from build123d import *

# Parameters (mm, degrees)
SKETCH1_R           = 59
BOSS_EXTRUDE1_DEPTH = 3
SKETCH3_R           = 51.75
BOSS_EXTRUDE2_DEPTH = 10
SKETCH4_R           = 50
CUT_EXTRUDE2_DEPTH  = 10
SCALE1_SCALE        = 0.5
SKETCH5_R           = 7.5
CUT_EXTRUDE3_DEPTH  = 15
SKETCH6_R           = 7.5
CUT_EXTRUDE4_DEPTH  = 15
SKETCH7_R           = 7.5
CUT_EXTRUDE5_DEPTH  = 15
SKETCH8_W           = 15
SKETCH8_H           = 16.086629849
CUT_EXTRUDE6_DEPTH  = 15


with BuildPart() as part:
    # Sketch1 → Boss-Extrude1 (new body)
    with BuildSketch(Plane(origin=(0, 0, 0), x_dir=(1, 0, 0), z_dir=(0, 1, 0))):
        with Locations(Location((0, 0, 0), (0, 0, 270))):
            Circle(SKETCH1_R)
    extrude(amount=BOSS_EXTRUDE1_DEPTH)

    # Sketch3 → Boss-Extrude2 (add)
    with BuildSketch(Plane(origin=(0, 3, 0), x_dir=(1, 0, 0), z_dir=(0, 1, 0))):
        with Locations(Location((0, 0, 0), (0, 0, 270))):
            Circle(SKETCH3_R)
    extrude(amount=BOSS_EXTRUDE2_DEPTH)

    # Sketch4 → Cut-Extrude2 (cut)
    with BuildSketch(Plane(origin=(0, 13, 0), x_dir=(1, 0, 0), z_dir=(0, 1, 0))):
        with Locations(Location((0, 0, 0), (0, 0, 270))):
            Circle(SKETCH4_R)
    extrude(amount=-CUT_EXTRUDE2_DEPTH, mode=Mode.SUBTRACT)


with BuildPart() as part_1:
    # Scale1: scaled about (0, 2.446860076, 0)
    add(part.part.scale(SCALE1_SCALE).moved(Location((0, 1.223430038, 0))))

    # Sketch5 → Cut-Extrude3 (cut)
    with BuildSketch(Plane(origin=(0, 2.723430038, 0), x_dir=(1, 0, 0), z_dir=(0, 1, 0))):
        with Locations(Location((0, -17.548132192, 0), (0, 0, 270))):
            Circle(SKETCH5_R)
    extrude(amount=-CUT_EXTRUDE3_DEPTH, mode=Mode.SUBTRACT)

    # Sketch6 → Cut-Extrude4 (cut)
    with BuildSketch(Plane(origin=(0, 7.723430038, 0), x_dir=(1, 0, 0), z_dir=(0, 1, 0))):
        with Locations((0, -25.513831206)):
            Circle(SKETCH6_R)
    extrude(amount=-CUT_EXTRUDE4_DEPTH, mode=Mode.SUBTRACT)

    # Sketch7 → Cut-Extrude5 (cut)
    with BuildSketch(Plane(origin=(0, 7.723430038, 0), x_dir=(1, 0, 0), z_dir=(0, 1, 0))):
        with Locations((0, -20.692487066)):
            Circle(SKETCH7_R)
    extrude(amount=-CUT_EXTRUDE5_DEPTH, mode=Mode.SUBTRACT)

    # Sketch8 → Cut-Extrude6 (cut)
    with BuildSketch(Plane(origin=(0, 2.723430038, 0), x_dir=(1, 0, 0), z_dir=(0, 1, 0))):
        with Locations((0, -25.591447116)):
            Rectangle(SKETCH8_W, SKETCH8_H)
    extrude(amount=-CUT_EXTRUDE6_DEPTH, mode=Mode.SUBTRACT)


solid = part_1.part
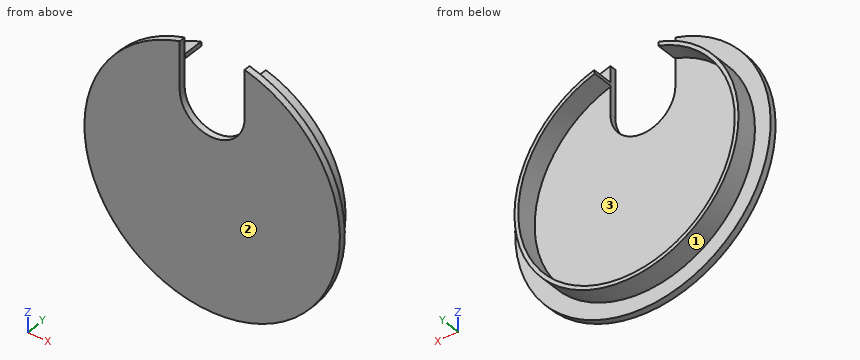
Input: part model. Units: mm. Frame: model coordinates. Face numbers are marked on the shaded views. Give positions to 0.01 mm unless a question says otherwise; leave off trailing zeros. Loops run counter-clockwise (first coordinate to the right, second up) from the corner with the lowest first, then second, coordinate; pieces in that order, holes last. Notation, with made-up numbers: M -35,10.5 L -29,10.5 A30 ccw -29,45.5 Z; hole C 57,85 d1. An arc over 180 degrees is marked long. Use one line per item in the form item = value.
1. Section query B-B, the plane x = -21. Return the cut outline in (y, z).
Numbers:
outline = M 1.22,-20.72 L 2.72,-20.72 L 2.72,-15.12 L 7.72,-15.12 L 7.72,-13.56 L 2.72,-13.56 L 2.72,13.56 L 7.72,13.56 L 7.72,15.12 L 2.72,15.12 L 2.72,20.72 L 1.22,20.72 Z
2. Section query A-A, the plane z = 12. Return the cut outline in (x, y), and give its area (3 significant figures).
Numbers:
outline = M -26.95,1.22 L -5.05,1.22 L -5.05,2.72 L -21.93,2.72 L -21.93,7.72 L -22.92,7.72 L -22.92,2.72 L -26.95,2.72 Z; M 5.05,1.22 L 26.95,1.22 L 26.95,2.72 L 22.92,2.72 L 22.92,7.72 L 21.93,7.72 L 21.93,2.72 L 5.05,2.72 Z
area = 75.6 mm²
3. Section query D-D, the plane y = 5. Return the cut outline in (x, z) (3 decimals).
Numbers:
outline = M -7.464,24.775 A25.875 ccw long 7.464,24.775 A7.5 cw 7.325,23.903 A25 cw long -7.325,23.903 A7.5 cw Z
4. First-contact query: pin 1 (1.5 mm diameter, centred on x = 11.5, y = 6, fed in from -Z); pin 2 (17.5 mm diameter, centred on x = 3, z = 14, fed in from +Y); pin 3 (1 mm diameter, centred on y = 5.5, z = 6, fed in from +X). Flat tips, straight axial feed; report the tip coordinate or a pass-through.
Numbers:
pin_1 = -23.54
pin_2 = 2.72
pin_3 = 25.28
5. Pull-direction query (X, two-part tool) for the marked faces 1, 2 and 3; classes: released by +X, released by -X, zero draft, split by the parting line, or undercut.
Numbers:
face_1 = split by the parting line
face_2 = zero draft
face_3 = undercut
6. Line query: L1, parallel to X at y = 6.45, z = 0 (3 decimals); L2, parallel to Z at x = 0, y = 5.25 (3 decimals); L3, parallel to Z at x = -12, y = 4.5. Output: solid intervals per line, ascending.
Numbers:
L1 = -25.875 to -25, 25 to 25.875
L2 = -25.875 to -25
L3 = -22.92 to -21.93, 21.93 to 22.92
7. Section query C-C, the plane z = 0. Return the cut outline in (x, y) (3 decimals), and give its area (4 significant figures).
Numbers:
outline = M -29.5,1.223 L 29.5,1.223 L 29.5,2.723 L 25.875,2.723 L 25.875,7.723 L 25,7.723 L 25,2.723 L -25,2.723 L -25,7.723 L -25.875,7.723 L -25.875,2.723 L -29.5,2.723 Z
area = 97.25 mm²
